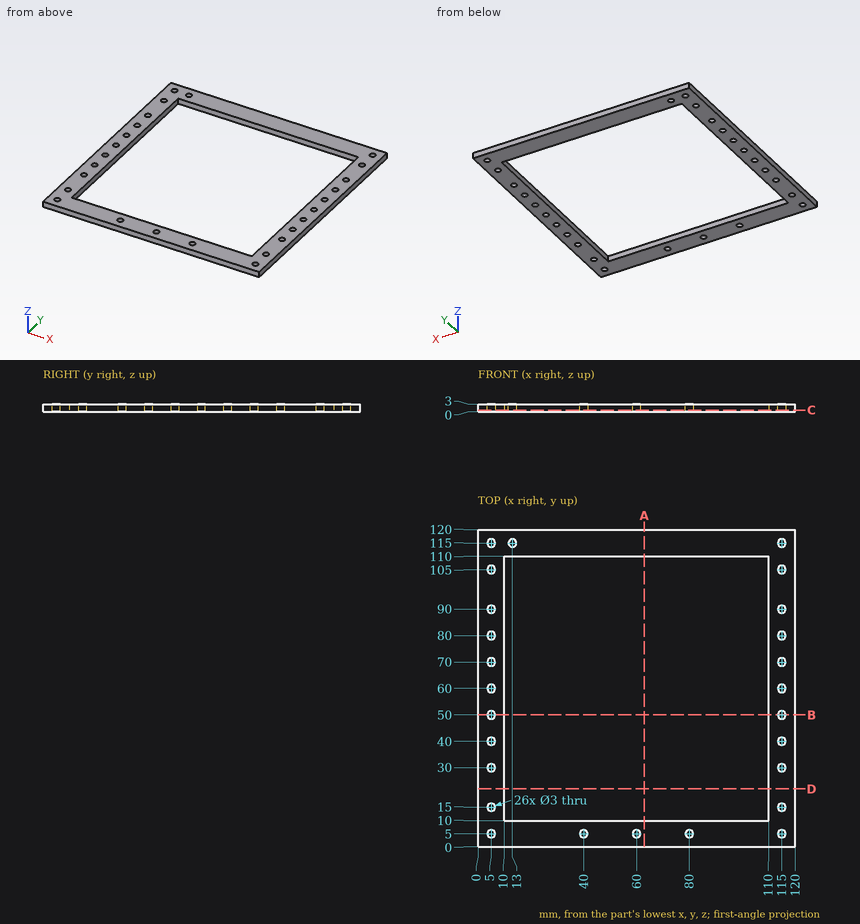
The figure shows three views and two pictorial views of one solid part (mm, origin at its lowest corner). Answer the questions. Give positions to 0.01 mm unless a question says otherwise; leave off trailing zeros. Order: outer loops, then holes, each group sorted by start corner. A loop starts at its lowest first (then second) coordinate and runs counter-clockwise, first axis right, second up. Notation, with made-up numbers: M 20,-33 L 73,-33 A22 cw 73,-9 Z; hole C 78,-27 d8. An arc over 180 degrees is marked long. Return JSON: item names as keys, results as strings.
Q1. Find section A-A, the plane x = 63. Write down the section's boundary in (y, z), and give its area (3 significant figures).
Answer below:
{"outline": "M 0,0 L 10,0 L 10,3 L 0,3 Z; M 110,0 L 120,0 L 120,3 L 110,3 Z", "area": "60.0 mm^2"}
Q2. Find section C-C, the plane z = 0.7. State how many separate pieces and enclosed holes the cut face has, and give its area (3 significant figures).
Answer below:
{"separate pieces": "1", "enclosed holes": "27", "area": "4,220 mm^2"}
Q3. Find the intervals of material crossed by line 1 along X through (y, z) = (70, 1.75); line 2 along X through (y, z) = (75, 0.35), in increasing order. Write a range as [from, to].
Answer below:
{"line 1": "x = [0, 3.5], [6.5, 10], [110, 113.5], [116.5, 120]", "line 2": "x = [0, 10], [110, 120]"}
Q4. Find section B-B, the plane y = 50. Write down the section's boundary in (x, z).
Answer below:
{"outline": "M 0,0 L 3.5,0 L 3.5,3 L 0,3 Z; M 6.5,0 L 10,0 L 10,3 L 6.5,3 Z; M 110,0 L 113.5,0 L 113.5,3 L 110,3 Z; M 116.5,0 L 120,0 L 120,3 L 116.5,3 Z"}
